Model file for the job. Use its own axes, mm. A direction names the side the tool comes from. Give positions to 0.01 mm unless a question says otherwise; leave off trailing zeros. Loops run counter-clockwise (first coordinate to the right, second up) from the corner with the lowest first, then second, coordinate; pieces in that order, holes last. Notation, with made-up numbers: (59.5, -11) -> (114.5, -11) arc R11 cw to (114.5, -5) -> close; hole circle Ø10 at (-32, 64). An arc over 180 degrees is marked (long way). Use CSV: the item, a comma, the result in double quotes. Start each with the question number.
(1) 3-axis set-ups, long thin cutter, end or side, ignore diameter. For faces 4 (the flat face through (-14, -12.954, 1)), 5 (the flat face through (-14, -3.81, 1)), 6 (the flat face through (8, 17.869, 1)), 7 (the flat face through (-4, 2, 0)), 8 (the flat face through (10, 1.321, 1)): which of +Z, -Z, +X, -X, +Y, -Y reach the whole face in a straight line?
(2) Cut at C-C on x = 0.5. Write the cut outline in (y, z).
(3) Cut at B-B on y = -3. Write the cut outline in (x, z).
(4) Flat gauge pins, fed straight in: pin 1 (8 mm diameter, centred on x = -14, y = 12, fed in from -Z); pin 2 (0.8 mm diameter, centred on y = 3, z = 1, fed in from +X) (3 decimals); pin 3 (0.5 mm diameter, centred on x = 10, z = 1, fed in from -Y); pin 4 (0.5 mm diameter, centred on x = -14.5, z = 1, fed in from +Y). Where does each tip first touch, or does it go through?
(5) Drill centre lines: probe 1 along Y at (x, z) = (8.5, 1); probe 2 along Y at (x, z) = (-11.5, 1.3); probe 3 along Y at (x, z) = (-5.08, 0.4). Where is each one in solid material? Low to high.
(6) Pull direction X, two halves, no side cores. Call faces 1 (the flat face through (-11.748, 2, 1)), 2 (the flat face through (10, -5.08, 1)), 3 (the cylindrical face through (-7.873, -8.462, 0.783)): pulls with the +X half, pulls with the -X half, needs draft (parallel to the pull), parting line crosses it, or undercut.
(7) Cut at A-A on x = -5.08. Write the cut outline in (y, z), then the cut area to 3 significant figures.
(8) Cut at D-D on x = -15. Write the cut outline in (y, z), then the cut area to 3 significant figures.
from build123d import *

# Parameters (mm, degrees)
SKETCH1_R           = 3.7592
BOSS_EXTRUDE1_DEPTH = 1.5875
CUT_EXTRUDE1_REACH  = 28.578
SKETCH2_W           = 3.302
SKETCH2_H           = 3.7592
CUT_EXTRUDE2_REACH  = 28.578
SKETCH3_W           = 8.3
SKETCH3_H           = 7.75
FILLET1_R           = 5.08
FILLET2_R           = 1.27


with BuildPart() as part:
    # Sketch1 → Boss-Extrude1 (new body)
    with BuildSketch(Plane.XY):
        with BuildLine():
            Line((11.1125, 17.8308), (9.525, 17.8308))
            Line((9.525, 17.8308), (9.525, 19.05))
            Line((9.525, 19.05), (2.54, 19.05))
            ThreePointArc((2.54, 19.05), (-6.440256121, 15.330256121), (-10.16, 6.35))
            Line((-10.16, 6.35), (-10.16, 2.5908))
            Line((-10.16, 2.5908), (-11.7475, 2.5908))
            Line((-11.7475, 2.5908), (-11.7475, 1.27))
            Line((-11.7475, 1.27), (-10.16, 1.27))
            Line((-10.16, 1.27), (-10.16, -3.81))
            Line((-10.16, -3.81), (-18.4658, -3.81))
            Line((-18.4658, -3.81), (-18.4658, -12.954))
            Line((-18.4658, -12.954), (-10.16, -12.954))
            Line((-10.16, -12.954), (-10.16, -14.859))
            Line((-10.16, -14.859), (9.525, -14.859))
            Line((9.525, -14.859), (9.525, -6.4008))
            Line((9.525, -6.4008), (11.1125, -6.4008))
            Line((11.1125, -6.4008), (11.1125, -5.08))
            Line((11.1125, -5.08), (9.525, -5.08))
            Line((9.525, -5.08), (9.525, 0))
            Line((9.525, 0), (11.1125, 0))
            Line((11.1125, 0), (11.1125, 1.3208))
            Line((11.1125, 1.3208), (9.525, 1.3208))
            Line((9.525, 1.3208), (9.525, 16.51))
            Line((9.525, 16.51), (11.1125, 16.51))
            Line((11.1125, 16.51), (11.1125, 17.8308))
        make_face()
        Circle(SKETCH1_R, mode=Mode.SUBTRACT)
        with BuildLine():
            ThreePointArc((-3.82905, -5.883688551), (4.572, -8.382), (-3.82905, -10.880311449))
            ThreePointArc((-3.82905, -10.880311449), (-7.874, -8.382), (-3.82905, -5.883688551))
        make_face(mode=Mode.SUBTRACT)
    extrude(amount=BOSS_EXTRUDE1_DEPTH)

    # Sketch2 → Cut-Extrude1 (cut, up to next)
    with BuildSketch(Plane.XY.offset(1.5875), mode=Mode.PRIVATE) as cut_extrude1_sk1:
        with Locations((7.874, -1.9685)):
            Rectangle(SKETCH2_W, SKETCH2_H)
    cut_extrude1_tool1 = extrude(cut_extrude1_sk1.sketch, amount=-CUT_EXTRUDE1_REACH, mode=Mode.PRIVATE) & part.part
    # Sketch2 → Cut-Extrude1 (cut, up to next)
    with BuildSketch(Plane.XY.offset(1.5875), mode=Mode.PRIVATE) as cut_extrude1_sk2:
        with Locations((7.874, 19.7485)):
            Rectangle(SKETCH2_W, SKETCH2_H)
    cut_extrude1_tool2 = extrude(cut_extrude1_sk2.sketch, amount=-CUT_EXTRUDE1_REACH, mode=Mode.PRIVATE) & part.part
    add(cut_extrude1_tool1.solids().sort_by_distance((7.874, -1.9685, 1.5875))[0], mode=Mode.SUBTRACT)
    add(cut_extrude1_tool2.solids().sort_by_distance((7.874, 19.7485, 1.5875))[0], mode=Mode.SUBTRACT)

    # Sketch3 → Cut-Extrude2 (cut, up to next)
    with BuildSketch(Plane(origin=(0, 0, 0), x_dir=(-1, 0, 0), z_dir=(0, 0, -1)), mode=Mode.PRIVATE) as cut_extrude2_sk1:
        with Locations((-8.3625, 8.656327373)):
            Rectangle(SKETCH3_W, SKETCH3_H)
    cut_extrude2_tool1 = extrude(cut_extrude2_sk1.sketch, amount=-CUT_EXTRUDE2_REACH, mode=Mode.PRIVATE) & part.part
    add(cut_extrude2_tool1.solids().sort_by_distance((8.3625, 8.656327, 0))[0], mode=Mode.SUBTRACT)

    # Fillet1
    fillet1_edges = [part.edges().sort_by_distance(p)[0] for p in [
        (9.525, -14.859, 0.79375),
    ]]
    fillet(fillet1_edges, radius=FILLET1_R)

    # Fillet2
    fillet2_edges = [part.edges().sort_by_distance(p)[0] for p in [
        (-10.16, -14.859, 0.79375),
    ]]
    fillet(fillet2_edges, radius=FILLET2_R)


solid = part.part
Check result:
1,face 4,"+Z, -Z, -X, -Y"
1,face 5,"+Z, -Z, -X"
1,face 6,"+Z, -Z, +X, +Y"
1,face 7,"-Z, +X, -X, +Y, -Y"
1,face 8,"+Z, -Z, +X"
2,outline,"(-14.86, 0) -> (-12.93, 0) -> (-12.93, 1.59) -> (-14.86, 1.59) -> close; (-3.84, 0) -> (-3.73, 0) -> (-3.73, 1.59) -> (-3.84, 1.59) -> close; (3.73, 0) -> (18.89, 0) -> (18.89, 1.59) -> (3.73, 1.59) -> close"
3,outline,"(-10.16, 0) -> (-2.27, 0) -> (-2.27, 1.59) -> (-10.16, 1.59) -> close; (2.27, 0) -> (6.22, 0) -> (6.22, 1.59) -> (2.27, 1.59) -> close"
4,pin 1,"through"
4,pin 2,"x = 9.525"
4,pin 3,"y = -6.4"
4,pin 4,"y = -3.81"
5,probe 1,"-12.84 to -3.85, -0.09 to 4.78, 12.53 to 17.87"
5,probe 2,"-12.95 to -3.81, 1.27 to 2.59"
5,probe 3,"-14.86 to -11.18, -5.59 to 16.51"
6,face 1,"pulls with the -X half"
6,face 2,"needs draft"
6,face 3,"undercut"
7,outline,"(-14.86, 0) -> (-11.18, 0) -> (-11.18, 1.59) -> (-14.86, 1.59) -> close; (-5.59, 0) -> (16.51, 0) -> (16.51, 1.59) -> (-5.59, 1.59) -> close"
7,area,"40.9 mm²"
8,outline,"(-12.95, 0) -> (-3.81, 0) -> (-3.81, 1.59) -> (-12.95, 1.59) -> close"
8,area,"14.5 mm²"
